The listing builds one solid part. Answer for the finished solid, in the listing's coordinates (mm). Face numbers are marked on the shaded views. A direction names the side the tool comes from. Round coordinates to 2 decimals unless told otherwise and drop trailing zeros. Write each loop counter-clockwise with the first axis right and the second up, starting at its lowest first coordinate (ties: lowest second). Pieces come first, ordered by that corner, then holes. Notation, with made-up numbers: (-25.75, 69.5) - (15.25, 69.5) arc R10 cw to (15.25, 79.5) - close; hole circle Ø5 at (-7, 19.25). An arc over 180 degrees is marked (long way). Return JSON: item names as keys, results as strings. Group by question number.
(1) Each of these flat-tipped pins is pushed along its axis until it touches: pin 1 (6 mm diameter, centred on x = 12, y = 11, fed in from -Z); pin 2 (4 mm diameter, centred on x = -4.5, y = 12.5, fed in from +Z); pin 3 (1.5 mm diameter, centred on x = 5, z = 76.5, fed in from -Y); pin 4 (4 mm diameter, centred on x = -14, y = -12, fed in from -Z). Where does it stop, or does it pass through?
(2) Which of the six approach directions +Z, -Z, +X, -X, +Y, -Y give full straight-line access (tool end or side, diameter ignored) to the marked faces 5, 6, 7, 8 and 9?
(3) Section B-B, the plane y = 8 is taken. Write down the section's boundary in (x, z).
(4) Section A-A, the plane z = 80 is taken. Write down the section's boundary in (x, y).
(5) Find the intervals of material crossed by line 1 along X through (y, z) = (-13.25, 40.7); line 2 along Z through (x, y) = (15.5, -17); line 3 along X through (y, z) = (-17, 40), in increasing order. Write a range as [from, to].
(6) Determine the mould class of the marked faces 1, 2, 3 and 4 for opening direction Y: +Y half, -Y half, draft (parallel to the pull), parting line (faces both ways), or undercut.
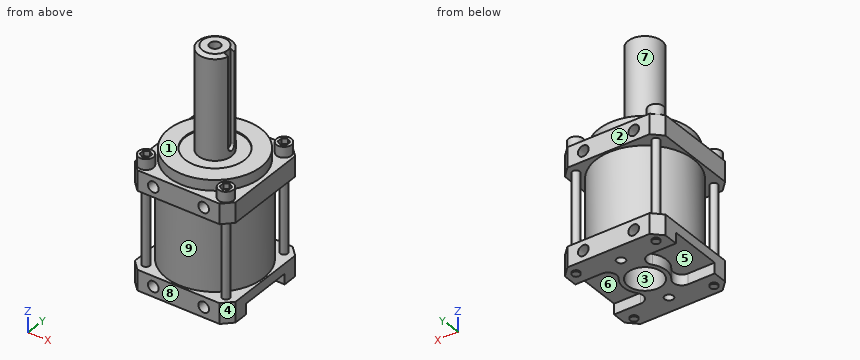
```python
from build123d import *

# Parameters (mm, degrees)
RESSALTO_EXTRUS_O1_DEPTH                      = 7.7
ESBO_O4_W                                     = 18.4
ESBO_O4_H                                     = 29.2
ESBO_O3_R                                     = 6.45
CORTE_EXTRUS_O1_DEPTH                         = 9.9
RESSALTO_EXTRUS_O2_DEPTH                      = 7.6
CORTE_EXTRUS_O2_DEPTH                         = 4
BROCA_DE_ROSQUEAR_PARA_TARRAXA_DE_10_32_D     = 4.0386
BROCA_DE_ROSQUEAR_PARA_TARRAXA_DE_10_32_DEPTH = 7.62
BROCA_DE_ROSQUEAR_PARA_TARRAXA_DE_10_32_TIP   = 1.213317848
ESBO_O9_W                                     = 1.795576077
ESBO_O9_H                                     = 3.175
CORTE_EXTRUS_O3_DEPTH                         = 36.5
FILETE1_R                                     = 1.58
BROCA_DE_ROSQUEAR_PARA_TARRAXA_DE_1_2_A_COUNT = 2
BROCA_DE_ROSQUEAR_PARA_TARRAXA_DE_1_2_A_PITCH = 19.05
BROCA_DE_ROSQUEAR_PARA_TARRAXA_DE_1_3_COUNT   = 2
BROCA_DE_ROSQUEAR_PARA_TARRAXA_DE_1_3_PITCH   = 41.482827772
BROCA_DE_ROSQUEAR_PARA_TARRAXA_DE_1_4_COUNT   = 2
BROCA_DE_ROSQUEAR_PARA_TARRAXA_DE_1_4_PITCH   = 36.85
BROCA_DE_ROSQUEAR_PARA_TARRAXA_DE_6_401_D     = 2.8702
CORTE_EXTRUS_O4_DEPTH                         = 2
ESPELHAR1_COPY_2_DEPTH                        = 2
ESCAREADO_PARA_PARAFUSO_DE_M_QUINA_C_2_COUNT  = 2
ESCAREADO_PARA_PARAFUSO_DE_M_QUINA_C_2_PITCH  = 25


with BuildPart() as part:
    # Esbo_o2 → Ressalto-extrus_o1 (new body)
    with BuildSketch(Plane.XY):
        Polygon((-19.03, 15.53), (-15.53, 19.03), (15.53, 19.03), (19.03, 15.53), (19.03, -15.53), (15.53, -19.03), (-15.53, -19.03), (-19.03, -15.53), align=None)
    extrude(amount=RESSALTO_EXTRUS_O1_DEPTH)

    # Esbo_o4 → Revolu_o1 (revolve)
    with BuildSketch(Plane(origin=(0, 0, 0), x_dir=(1, 0, 0), z_dir=(0, 1, 0)), mode=Mode.PRIVATE) as revolu_o1_sk:
        with Locations((9.2, -22.3)):
            Rectangle(ESBO_O4_W, ESBO_O4_H)
        Polygon((0, -44.5), (17.5, -44.5), (17.5, -48.5), (11.2, -48.5), (11.2, -48), (6.35, -48), (6.35, -85.576239569), (4.75, -86.5), (0, -86.5), align=None)
    revolve(revolu_o1_sk.sketch.rotate(Axis((0, 0, -5.757774852), (0, 0, 1)), 180), axis=Axis((0, 0, -5.757774852), (0, 0, 1)))


with BuildPart() as revolu_o1_piece_1:
    # of the separate pieces the step leaves, piece 1, a body of its own (revolu_o1_pieces)
    add(part.part.solids().sort_by_distance((-19.03, 15.53, 0))[0])

    # Esbo_o3 → Corte-extrus_o1 (cut)
    with BuildSketch(Plane(origin=(0, 0, 0), x_dir=(-1, 0, 0), z_dir=(0, 0, -1))):
        Circle(ESBO_O3_R)
    extrude(amount=-CORTE_EXTRUS_O1_DEPTH, mode=Mode.SUBTRACT)



with BuildPart() as revolu_o1_piece_2:
    # of the separate pieces the step leaves, piece 2, a body of its own (revolu_o1_pieces)
    add(part.part.solids().sort_by_distance((-17.5, 0, 44.5))[0])


with BuildPart() as revolu_o1_piece_1_1:
    add(revolu_o1_piece_1.part)

    add(revolu_o1_piece_2.part)  # Ressalto-extrus_o2 merges Revolu_o1 piece 2
    # Esbo_o5 → Ressalto-extrus_o2 (add)
    with BuildSketch(Plane.XY.offset(36.9)):
        Polygon((-15.53, 19.03), (-19.03, 15.53), (-19.03, -15.53), (-15.53, -19.03), (15.53, -19.03), (19.03, -15.53), (19.03, 15.53), (15.53, 19.03), align=None)
    extrude(amount=RESSALTO_EXTRUS_O2_DEPTH)

    # Esbo_o6 → Corte-extrus_o2 (cut)
    with BuildSketch(Plane(origin=(0, 0, 0), x_dir=(-1, 0, 0), z_dir=(0, 0, -1))):
        with BuildLine():
            Line((-19.03, -10.1), (-19.03, 10.1))
            Line((-19.03, 10.1), (-9.012713751, 10.1))
            ThreePointArc((-9.012713751, 10.1), (-6.090453498, 8.288387911), (-6.413345842, 4.865336074))
            ThreePointArc((-6.413345842, 4.865336074), (-8.05, 0), (-6.413345842, -4.865336074))
            ThreePointArc((-6.413345842, -4.865336074), (-6.090453498, -8.288387911), (-9.012713751, -10.1))
            Line((-9.012713751, -10.1), (-19.03, -10.1))
        make_face()
        with BuildLine():
            Line((19.03, -10.1), (9.012713751, -10.1))
            ThreePointArc((9.012713751, -10.1), (6.090453498, -8.288387911), (6.413345842, -4.865336074))
            ThreePointArc((6.413345842, -4.865336074), (8.05, 0), (6.413345842, 4.865336074))
            ThreePointArc((6.413345842, 4.865336074), (6.090453498, 8.288387911), (9.012713751, 10.1))
            Line((9.012713751, 10.1), (19.03, 10.1))
            Line((19.03, 10.1), (19.03, -10.1))
        make_face()
    extrude(amount=-CORTE_EXTRUS_O2_DEPTH, mode=Mode.SUBTRACT)

    # Broca de rosquear para tarraxa de _10-32
    with Locations(Plane.XY.offset(86.5)):
        with Locations((0, 0)):
            Hole(BROCA_DE_ROSQUEAR_PARA_TARRAXA_DE_10_32_D / 2, depth=BROCA_DE_ROSQUEAR_PARA_TARRAXA_DE_10_32_DEPTH)
            with Locations((0, 0, -(BROCA_DE_ROSQUEAR_PARA_TARRAXA_DE_10_32_DEPTH + BROCA_DE_ROSQUEAR_PARA_TARRAXA_DE_10_32_TIP / 2))):  # 118° drill point
                Cone(0, BROCA_DE_ROSQUEAR_PARA_TARRAXA_DE_10_32_D / 2, BROCA_DE_ROSQUEAR_PARA_TARRAXA_DE_10_32_TIP, mode=Mode.SUBTRACT)

    # Esbo_o9 → Corte-extrus_o3 (cut)
    with BuildSketch(Plane.XY.offset(86.5)):
        with Locations((5.647788038, 0)):
            Rectangle(ESBO_O9_W, ESBO_O9_H)
    extrude(amount=-CORTE_EXTRUS_O3_DEPTH, mode=Mode.SUBTRACT)

    # Filete1
    filete1_edges = [revolu_o1_piece_1_1.edges().sort_by_distance(p)[0] for p in [
        (5.449180531, 1.5875, 50),
        (5.449180531, -1.5875, 50),
    ]]
    fillet(filete1_edges, radius=FILETE1_R)

    # Esbo_o11 → Broca de rosquear para tarraxa de _1 2 (revolve, cut)
    with BuildSketch(Plane(origin=(9.525, 19.03, 3.85), x_dir=(0, 0, 1), z_dir=(1, 0, 0))):
        Polygon((0, 0), (0, 8.833317848), (2.0193, 7.62), (2.0193, 0), align=None)
    broca_de_rosquear_para_tarraxa_de_1_2 = revolve(axis=Axis((9.525, 25.38, 3.85), (0, -1, 0)), mode=Mode.SUBTRACT)

    # Broca de rosquear para tarraxa de _1 2 a: Broca de rosquear para tarraxa de _1 2 ×2
    with Locations(*[(-i * BROCA_DE_ROSQUEAR_PARA_TARRAXA_DE_1_2_A_PITCH, 0, 0) for i in range(1, BROCA_DE_ROSQUEAR_PARA_TARRAXA_DE_1_2_A_COUNT)]):
        add(broca_de_rosquear_para_tarraxa_de_1_2, mode=Mode.SUBTRACT)

    # Broca de rosquear para tarraxa de _1 3: Broca de rosquear para tarraxa de _1 2 ×2
    with Locations(*[Vector(-0.45922616713812264, 0, 0.8883193836766308) * (i * BROCA_DE_ROSQUEAR_PARA_TARRAXA_DE_1_3_PITCH) for i in range(1, BROCA_DE_ROSQUEAR_PARA_TARRAXA_DE_1_3_COUNT)]):
        add(broca_de_rosquear_para_tarraxa_de_1_2, mode=Mode.SUBTRACT)

    # Broca de rosquear para tarraxa de _1 4: Broca de rosquear para tarraxa de _1 2 ×2
    with Locations(*[(0, 0, i * BROCA_DE_ROSQUEAR_PARA_TARRAXA_DE_1_4_PITCH) for i in range(1, BROCA_DE_ROSQUEAR_PARA_TARRAXA_DE_1_4_COUNT)]):
        add(broca_de_rosquear_para_tarraxa_de_1_2, mode=Mode.SUBTRACT)

    # Espelhar3: Broca de rosquear para tarraxa de _1 2 across plane
    add(broca_de_rosquear_para_tarraxa_de_1_2.mirror(Plane.ZX), mode=Mode.SUBTRACT)

    # Espelhar3 copy 1 sketch → Espelhar3 copy 1 (revolve, cut)
    with BuildSketch(Plane(origin=(-9.525, -19.03, 3.85), x_dir=(0, 0, 1), z_dir=(1, 0, 0))):
        Polygon((0, 0), (0, -8.833317848), (2.0193, -7.62), (2.0193, 0), align=None)
    revolve(axis=Axis((-9.525, -25.38, 3.85), (0, -1, 0)), mode=Mode.SUBTRACT)

    # Espelhar3 copy 2 sketch → Espelhar3 copy 2 (revolve, cut)
    with BuildSketch(Plane(origin=(-9.525, -19.03, 40.7), x_dir=(0, 0, 1), z_dir=(1, 0, 0))):
        Polygon((0, 0), (0, -8.833317848), (2.0193, -7.62), (2.0193, 0), align=None)
    revolve(axis=Axis((-9.525, -25.38, 40.7), (0, -1, 0)), mode=Mode.SUBTRACT)

    # Espelhar3 copy 3 sketch → Espelhar3 copy 3 (revolve, cut)
    with BuildSketch(Plane(origin=(9.525, -19.03, 40.7), x_dir=(0, 0, 1), z_dir=(1, 0, 0))):
        Polygon((0, 0), (0, -8.833317848), (2.0193, -7.62), (2.0193, 0), align=None)
    revolve(axis=Axis((9.525, -25.38, 40.7), (0, -1, 0)), mode=Mode.SUBTRACT)

    # Broca de rosquear para tarraxa de _6-401 (through all)
    with Locations(Plane(origin=(0, 0, 0), x_dir=(-1, 0, 0), z_dir=(0, 0, -1))):
        with Locations((-15.115, 15.115), (15.115, 15.115), (15.115, -15.115), (-15.115, -15.115)):
            Hole(BROCA_DE_ROSQUEAR_PARA_TARRAXA_DE_6_401_D / 2)

    # Esbo_o16 → Revolu_o2 (revolve)
    with BuildSketch(Plane(origin=(0, 15.115, 0), x_dir=(1, 0, 0), z_dir=(0, 1, 0))):
        Polygon((15.115, 0.5), (16.5501, 0.5), (16.5501, -44.5), (17.95, -44.5), (17.95, -48.5), (15.115, -48.5), align=None)
    revolu_o2 = revolve(axis=Axis((15.115, 15.115, 60.999619422), (0, 0, -1)))

    # Esbo_o17 → Corte-extrus_o4 (cut)
    with BuildSketch(Plane.XY.offset(48.5)):
        Polygon((13.410197167, 16.099268375), (13.410197167, 14.130731625), (15.115, 13.146463251), (16.819802833, 14.130731625), (16.819802833, 16.099268375), (15.115, 17.083536749), align=None)
    corte_extrus_o4 = extrude(amount=-CORTE_EXTRUS_O4_DEPTH, mode=Mode.SUBTRACT)

    # Espelhar2: Revolu_o2, Corte-extrus_o4 across plane
    add(revolu_o2.mirror(Plane(origin=(0, 0, 0), x_dir=(0, 0, 1), z_dir=(1, 0, 0))))
    add(corte_extrus_o4.mirror(Plane(origin=(0, 0, 0), x_dir=(0, 0, 1), z_dir=(1, 0, 0))), mode=Mode.SUBTRACT)

    # Espelhar1: Revolu_o2, Corte-extrus_o4 across plane
    add(revolu_o2.mirror(Plane.ZX))
    add(corte_extrus_o4.mirror(Plane.ZX), mode=Mode.SUBTRACT)

    # Espelhar1 copy 1 sketch → Espelhar1 copy 1 (revolve)
    with BuildSketch(Plane(origin=(0, -15.115, 0), x_dir=(-1, 0, 0), z_dir=(0, -1, 0))):
        Polygon((15.115, 0.5), (16.5501, 0.5), (16.5501, -44.5), (17.95, -44.5), (17.95, -48.5), (15.115, -48.5), align=None)
    revolve(axis=Axis((-15.115, -15.115, 60.999619422), (0, 0, -1)))

    # Espelhar1 copy 2 sketch → Espelhar1 copy 2 (cut)
    with BuildSketch(Plane(origin=(0, 0, 48.5), x_dir=(-1, 0, 0), z_dir=(0, 0, 1))):
        Polygon((13.410197167, 16.099268375), (13.410197167, 14.130731625), (15.115, 13.146463251), (16.819802833, 14.130731625), (16.819802833, 16.099268375), (15.115, 17.083536749), align=None)
    extrude(amount=-ESPELHAR1_COPY_2_DEPTH, mode=Mode.SUBTRACT)

    # Esbo_o19 → Escareado para parafuso de m_quina com c (revolve, cut)
    with BuildSketch(Plane(origin=(0, 12.5, 7.7), x_dir=(0, -1, 0), z_dir=(1, 0, 0))):
        Polygon((0, 0), (0, 8.2), (1.63195, 8.2), (1.63195, 1.804295328), (3.2004, 0), align=None)
    escareado_para_parafuso_de_m_quina_com_c = revolve(axis=Axis((0, 12.5, 14.05), (0, 0, -1)), mode=Mode.SUBTRACT)

    # Escareado para parafuso de m_quina c 2: Escareado para parafuso de m_quina com c ×2
    with Locations(*[(0, -i * ESCAREADO_PARA_PARAFUSO_DE_M_QUINA_C_2_PITCH, 0) for i in range(1, ESCAREADO_PARA_PARAFUSO_DE_M_QUINA_C_2_COUNT)]):
        add(escareado_para_parafuso_de_m_quina_com_c, mode=Mode.SUBTRACT)


solid = revolu_o1_piece_1_1.part
```
Working result:
{
 "1": {"pin 1": "stops at z = 0", "pin 2": "stops at z = 48.5", "pin 3": "stops at y = -4.72", "pin 4": "stops at z = -0.5"},
 "2": {"face 5": "-Z, -X", "face 6": "-Z, +X", "face 7": "+Z", "face 8": "+Z, -Z, +X, -X, -Y", "face 9": "none"},
 "3": {"outline": "(-19.03, 4) - (-5.96, 4) - (-5.96, 0) - (5.96, 0) - (5.96, 4) - (19.03, 4) - (19.03, 7.7) - (16.57, 7.7) - (16.57, 36.9) - (19.03, 36.9) - (19.03, 44.5) - (15.56, 44.5) - (15.56, 48.5) - (7.84, 48.5) - (7.84, 48) - (-7.84, 48) - (-7.84, 48.5) - (-15.56, 48.5) - (-15.56, 44.5) - (-19.03, 44.5) - (-19.03, 36.9) - (-16.57, 36.9) - (-16.57, 7.7) - (-19.03, 7.7) - close"},
 "4": {"outline": "(4.75, -1.59) - (4.75, 1.59) - (6.15, 1.59) arc R6.35 ccw (long way) to (6.15, -1.59) - close; hole circle Ø4.04 at (0, 0)"},
 "5": {"line 1": "x = [-19.03, -11.54], [-7.51, 7.51], [11.54, 19.03]", "line 2": "z = [0, 7.7], [36.9, 48.5]", "line 3": "x = [-17.56, -11.42], [-7.63, 7.63], [11.42, 17.56]"},
 "6": {"face 1": "draft", "face 2": "+Y half", "face 3": "undercut", "face 4": "-Y half"}
}
